Model file for the job. Use its own axes, mm. Face numbers are marked on the shaded views. A direction names the side the tool comes from. Round coordinates to 2 decimals unless told otherwise and drop trailing zeros. Loops run counter-clockwise (first coordinate to the right, second up) from the corner with the lowest first, then second, coordinate; pieces in that order, holes last. Notation, with made-up numbers: M 61,5.5 L 84,5.5 A22 ccw 84,25.5 Z; hole C -26.75,-29 d2. An arc over 180 degrees is marked long. Use a Markdown table: item, result. Add a question column.
Q1. Cut at C-C (z = 7.5). Give the cut face in (x, y), plus the area to 3 significant figures.
Q2. Probe line 1 (Z direction, x = 5, y = -16); line 2 (Y direction, x = -4.75, z = 7.5); line 3 (Z direction, x = -7.25, y = 11). List the from-to ranges inside material, lowest first. Write a range as from..to.
Q3. Pin check, flat tips, straight feed: pin 1 (3 mm diameter, centred on y = 21, z = 9.5, fed in from +X); pin 2 (1.6 mm diameter, centred on x = -6, z = 11, fed in from -Y). Stop position of each tip, or through.
Q4. Cut at B-B (x = 5). Give the cut face in (y, z), plus the area to 3 significant figures.
Q5. Cut at D-D (z = 4.5). Give the cut face in (x, y), plus the area to 3 significant figures.
Q6. Tool access for the marked faces 1 and 2: list every direction of +Z, -Z, +X, -X, +Y, -Y with a clear straight run to the whole face (end or side of a thin tool).
Q7. Cut at A-A (y = 55). Give the cut face in (x, z), plus the area to 3 significant figures.
from build123d import *

# Parameters (mm, degrees)
BOSS_EXTRUDE1_DEPTH = 15
FILLET1_R           = 5
SKETCH2_W           = 10
SKETCH2_H           = 15
BOSS_EXTRUDE2_DEPTH = 40
SKETCH3_R           = 2
CUT_EXTRUDE1_DEPTH  = 81
CUT_EXTRUDE2_DEPTH  = 11
SKETCH5_R           = 2
CUT_EXTRUDE3_DEPTH  = 21


with BuildPart() as part:
    # Sketch1 → Boss-Extrude1 (new body)
    with BuildSketch(Plane.XY):
        Polygon((0, 20), (0, -10), (10, -10), (10, -20), (-10, -20), (-10, 20), align=None)
    extrude(amount=BOSS_EXTRUDE1_DEPTH)

    # Fillet1
    fillet1_edges = [part.edges().sort_by_distance(p)[0] for p in [
        (-10, -20, 7.5),
    ]]
    fillet(fillet1_edges, radius=FILLET1_R)

    # Sketch2 → Boss-Extrude2 (add)
    with BuildSketch(Plane(origin=(0, 20, 0), x_dir=(1, 0, 0), z_dir=(0, 1, 0))):
        with Locations((-5, -7.5)):
            Rectangle(SKETCH2_W, SKETCH2_H)
    extrude(amount=BOSS_EXTRUDE2_DEPTH)

    # Sketch3 → Cut-Extrude1 (cut, through all)
    with BuildSketch(Plane.XZ.offset(20)):
        with Locations((5, 7.5)):
            Circle(SKETCH3_R)
    extrude(amount=-CUT_EXTRUDE1_DEPTH, mode=Mode.SUBTRACT)

    # Sketch4 → Cut-Extrude2 (cut, through all)
    with BuildSketch(Plane(origin=(0, 0, 0), x_dir=(0, 0, -1), z_dir=(1, 0, 0))):
        with BuildLine():
            Line((-10.48, 10), (-11.98, 10))
            ThreePointArc((-11.98, 10), (-13.040660172, 10.439339828), (-13.48, 11.5))
            Line((-13.48, 11.5), (-13.48, 12.5))
            ThreePointArc((-13.48, 12.5), (-13.040660172, 13.560660172), (-11.98, 14))
            Line((-11.98, 14), (-10.48, 14))
            ThreePointArc((-10.48, 14), (-9.419339828, 13.560660172), (-8.98, 12.5))
            Line((-8.98, 12.5), (-8.98, 11.5))
            ThreePointArc((-8.98, 11.5), (-9.419339828, 10.439339828), (-10.48, 10))
        make_face()
    extrude(amount=-CUT_EXTRUDE2_DEPTH, mode=Mode.SUBTRACT)

    # Sketch5 → Cut-Extrude3 (cut, through all)
    with BuildSketch(Plane.ZY.offset(10)):
        with Locations((7.5, 55)):
            Circle(SKETCH5_R)
    extrude(amount=-CUT_EXTRUDE3_DEPTH, mode=Mode.SUBTRACT)


solid = part.part
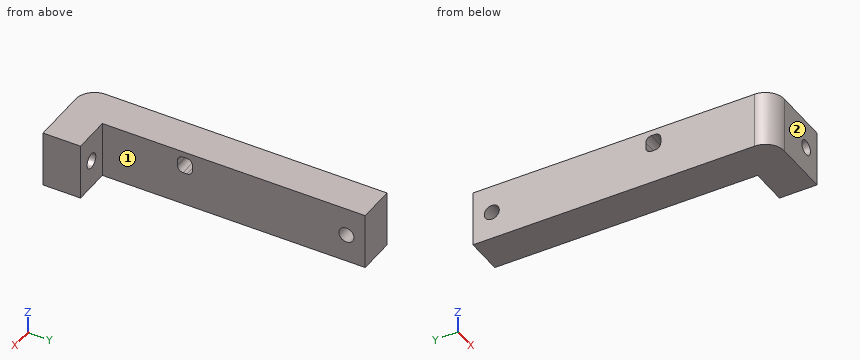
Checked values:
| question | item | result |
|---|---|---|
| 1 | outline | M -10,-15 A5 ccw -5,-20 L 3,-20 L 3,-10 L 0,-10 L 0,53 L -10,53 Z; M -10,57 L 0,57 L 0,60 L -10,60 Z; M 7,-20 L 10,-20 L 10,-10 L 7,-10 Z |
| 1 | area | 815 mm^2 |
| 2 | line 1 | z = 0..5.5, 9.5..15 |
| 2 | line 2 | y = -20..53, 57..60 |
| 2 | line 3 | z = 0..9.07, 13.39..15 |
| 3 | pin 1 | stops at x = 0 |
| 3 | pin 2 | stops at y = -20 |
| 4 | outline | M -20,0 L -10,0 L -10,5.5 L -20,5.5 Z; M -20,9.5 L -10,9.5 L -10,15 L -20,15 Z |
| 4 | area | 110 mm^2 |
| 5 | outline | M -10,-15 A5 ccw -5,-20 L 10,-20 L 10,-10 L 0,-10 L 0,60 L -10,60 Z |
| 5 | area | 895 mm^2 |
| 6 | face 1 | +Z, -Z, +X, +Y |
| 6 | face 2 | +Z, -Z, +X, -X, -Y |
| 7 | outline | M -10,0 L 0,0 L 0,5.5 L -10,5.5 Z; M -10,9.5 L 0,9.5 L 0,15 L -10,15 Z |
| 7 | area | 110 mm^2 |
